Autodesk Fusion 360 part; units mm, degrees
sketch "スケッチ1" plane through (0, 0, 0) normal (0, 0, 1) x (1, 0, 0)
  circle A0 centre (0, 0) radius 23
  circle A1 centre (0, 0) radius 21.25
  dimension "d1" = 46
  dimension "d2" = 42.5
extrude "押し出し1" add sketch "スケッチ1" along normal blind 2 contours A1
extrude "押し出し2" add sketch "スケッチ1" along normal blind 9
sketch "スケッチ2" plane through (0, 0, 0) normal (0, 0, -1) x (1, 0, 0)
  circle A0 centre (0, 0) radius 23
  circle A1 centre (0, 0) radius 13
  dimension "d7" = 26
extrude "押し出し3" cut sketch "スケッチ2" against normal blind 3 contours A1
sketch "スケッチ3" plane through (0, 0, 0) normal (0, 0, -1) x (1, 0, 0)
  circle A0 centre (0, 0) radius 13
  circle A1 centre (0, 0) radius 23
  line L0 (18.1, -11.26) -> (-18.1, -11.26)
  line L1 (-18.1, -11.26) -> (-18.1, 14.3567)
  line L2 (-18.1, 14.3567) -> (18.1, 14.3567)
  line L3 (18.1, 14.3567) -> (18.1, -11.26)
  line L4 (19.3, -12.3) -> (-19.3, -12.3)
  line L5 (-19.3, -12.3) -> (-19.3, 12.4)
  line L6 (-19.3, 12.4) -> (19.3, 12.4)
  line L7 (19.3, 12.4) -> (19.3, -12.3)
  dimension "d10" = 11.26
  dimension "d11" = 18.1
  dimension "d12" = 18.1
  dimension "d13" = 12.3
  dimension "d14" = 19.3
  dimension "d15" = 19.3
  dimension "d16" = 12.4
extrude "押し出し4" add sketch "スケッチ3" along normal blind 12 contours A0 L0 L3 L4 L6 L7 | A0 L0 L4 | A0 L0 L1 L4 L5 L6
sketch "スケッチ4" plane through (0, 0, 0) normal (0, 0, 1) x (-1, 0, 0)
  arc A0 (4.2083, -12.3) -> (6.4971, -11.26) centre (0, 0) ccw
  line L0 (6.4971, -11.26) -> (-6.4971, -11.26)
  arc A1 (-6.4971, -11.26) -> (-4.2083, -12.3) centre (0, 0) ccw
  line L1 (-4.2083, -12.3) -> (4.2083, -12.3)
  line L2 (8.6335, -10.0758) -> (-7.7138, -10.0758)
  line L3 (-7.7138, -10.0758) -> (-7.7138, -15.2171)
  line L4 (-7.7138, -15.2171) -> (8.6335, -15.2171)
  line L5 (8.6335, -15.2171) -> (8.6335, -10.0758)
  circle A2 centre (0, 0) radius 13
  circle A3 centre (0, 0) radius 14
  line L6 (9.1438, -11.26) -> (-8.6053, -11.26)
  dimension "d19" = 26
  dimension "d20" = 28
extrude "押し出し5" add sketch "スケッチ4" against normal blind 2 contours L1 A2 | A0 A1 L3 A2 A3 L6
Input: part model. Units: mm. Frame: model coordinates. A direction names the side the tool comes from. Coordinates: 2 decimals unless noted, no trailing zeros. Loops run counter-clockwise (first coordinate to the right, second up) from the corner with the lowest first, then second, coordinate; pieces in that order, holes last. Notation, with made-up numbers: (-38, 86.25) - (-10, 86.25) arc R12 cw to (-10, 99.25) - close; hole circle Ø4 at (24.5, 56). An arc over 180 degrees is marked (long way). Answer in a Markdown table with one row per item. Add a question column.
Item 1: Section query B-B on x = 0. Return the cut outline in (y, z).
Item 2: Section query D-D on x = 8. Return the cut outline in (y, z), then the cut area to 3 significant figures.
Item 3: Mould query, pull axis Y, two halves, no side actions, for faces 1 (the flat face through (0, 12, 0)), 2 (the cylindrical face through (0, 14, -1)), 3 (the flat face through (19.3, 0, -6)), 4 (the flat face through (-10, -9, 2)). Classes: released by +Y, released by -Y, zero draft, split by the parting line, or undercut.
Item 4: Line query: line 1 along X through (y, z) = (-8.5, -1.25); line 2 along Y through (x, z) = (0, 3.5); line 3 along Y through (x, z) = (-17, -10.25). Output: solid intervals per line, ascending. Write a range as [from, to].
Item 5: Section query A-A on y = 0. Return the cut outline in (x, z).
Item 6: Contact query for flat-ended pins moving along their axis: P1, Ø0.6, axis at x = -18.5, z = -7.5, coming from the -Y side; P2, Ø6, axis at y = -5.5, z = -6.5, coming from the +X side; P3, Ø14, axis at x = -2.5, y = -10.5, coming from the -Z side. Output: stop coordinate, or through.
Item 7: Section query C-C on z = 4.75. Return the cut outline in (x, y), then the cut area to 3 significant figures.
Item 8: Access query for faces 5 (the flat face through (0, 11.26, -6)), 6 (the cylindrical face through (-16.863, 12.93, 5.451)), 7 (the flat face through (19, -12.4, -6)). Directions: +Z, -Z, +X, -X, +Y, -Y. A direction counts if a zero-diameter tool reaches every point of the face in a straight line with its end or side. Return the directions, or none.
Recorded:
| question | item | result |
|---|---|---|
| 1 | outline | (-23, 0) - (-13, 0) - (-13, 2) - (-21.25, 2) - (-21.25, 9) - (-23, 9) - close; (11.26, -12) - (12.3, -12) - (12.3, -2) - (14, -2) - (14, 0) - (23, 0) - (23, 9) - (21.25, 9) - (21.25, 2) - (13, 2) - (13, 0) - (11.26, 0) - close |
| 2 | outline | (-21.56, 0) - (-10.25, 0) - (-10.25, 2) - (-19.69, 2) - (-19.69, 9) - (-21.56, 9) - close; (10.25, 0) - (11.26, 0) - (11.26, -12) - (12.3, -12) - (12.3, 0) - (21.56, 0) - (21.56, 9) - (19.69, 9) - (19.69, 2) - (10.25, 2) - close |
| 2 | area | 84.0 mm^2 |
| 3 | face 1 | undercut |
| 3 | face 2 | released by +Y |
| 3 | face 3 | zero draft |
| 3 | face 4 | undercut |
| 4 | line 1 | [-19.3, -18.1], [18.1, 19.3] |
| 4 | line 2 | [-23, -21.25], [21.25, 23] |
| 4 | line 3 | [11.26, 12.3] |
| 5 | outline | (-23, 0) - (-19.3, 0) - (-19.3, -12) - (-18.1, -12) - (-18.1, 0) - (-13, 0) - (-13, 2) - (-21.25, 2) - (-21.25, 9) - (-23, 9) - close; (13, 0) - (18.1, 0) - (18.1, -12) - (19.3, -12) - (19.3, 0) - (23, 0) - (23, 9) - (21.25, 9) - (21.25, 2) - (13, 2) - close |
| 6 | P1 | y = -12.4 |
| 6 | P2 | x = 19.3 |
| 6 | P3 | z = 0 |
| 7 | outline | circle Ø46 at (0, 0); hole circle Ø42.5 at (0, 0) |
| 7 | area | 243 mm^2 |
| 8 | face 5 | -Z, -Y |
| 8 | face 6 | +Z |
| 8 | face 7 | -Z, +X, -X, -Y |
